```python
from build123d import *

# Parameters (mm, degrees)
SKETCH_1_R      = 2.125
SKETCH_1_R_2    = 8
EXTRUDE_1_DEPTH = 6


with BuildPart() as part:
    # 草图1 → 凸台-拉伸1 (new body)
    with BuildSketch(Plane.XY):
        with BuildLine():
            Line((-22.390026272, -12.434766873), (21.159720544, -12.434766873))
            ThreePointArc((21.159720544, -12.434766873), (27.298604017, -11.469317294), (32.844809242, -8.666177844))
            Line((32.844809242, -8.666177844), (77.295062426, 23.333822156))
            ThreePointArc((77.295062426, 23.333822156), (83.410279539, 30.44661958), (85.609973728, 39.565233127))
            Line((85.609973728, 39.565233127), (85.609973728, 149.565233127))
            Line((85.609973728, 149.565233127), (35.609973728, 149.565233127))
            Line((35.609973728, 149.565233127), (35.609973728, 39.565233127))
            Line((35.609973728, 39.565233127), (27.609973728, 39.565233127))
            Line((27.609973728, 39.565233127), (-22.390026272, 39.565233127))
            Line((-22.390026272, 39.565233127), (-22.390026272, -12.434766873))
        make_face()
        with Locations((-12.390026272, -2.434766873)):
            Circle(SKETCH_1_R, mode=Mode.SUBTRACT)
        with Locations((-4.390026272, -2.434766873)):
            Circle(SKETCH_1_R, mode=Mode.SUBTRACT)
        with Locations((19.609973728, -2.434766873)):
            Circle(SKETCH_1_R, mode=Mode.SUBTRACT)
        with Locations((-12.390026272, 29.565233127)):
            Circle(SKETCH_1_R, mode=Mode.SUBTRACT)
        with Locations((-4.390026272, 29.565233127)):
            Circle(SKETCH_1_R, mode=Mode.SUBTRACT)
        with Locations((19.609973728, 29.565233127)):
            Circle(SKETCH_1_R, mode=Mode.SUBTRACT)
        with Locations((3.609973728, 13.565233127)):
            Circle(SKETCH_1_R_2, mode=Mode.SUBTRACT)
        with BuildLine():
            Line((54.859973728, 92.565233127), (54.859973728, 62.565233127))
            ThreePointArc((54.859973728, 62.565233127), (50.609973728, 58.315233127), (46.359973728, 62.565233127))
            Line((46.359973728, 62.565233127), (46.359973728, 92.565233127))
            ThreePointArc((46.359973728, 92.565233127), (50.609973728, 96.815233127), (54.859973728, 92.565233127))
        make_face(mode=Mode.SUBTRACT)
        with BuildLine():
            Line((66.359973728, 109.565233127), (66.359973728, 139.565233127))
            ThreePointArc((66.359973728, 139.565233127), (70.609973728, 143.815233127), (74.859973728, 139.565233127))
            Line((74.859973728, 139.565233127), (74.859973728, 109.565233127))
            ThreePointArc((74.859973728, 109.565233127), (70.609973728, 105.315233127), (66.359973728, 109.565233127))
        make_face(mode=Mode.SUBTRACT)
    extrude(amount=EXTRUDE_1_DEPTH)


solid = part.part
```
Design review of the part built by this model. Coordinates are the model's own, in mm. A direction names the side the tool comes from. Round coordinates to 2 decimals unless told otherwise and drop trailing zeros. Order: outer loops, then holes, each group sorted by start corner. A loop starts at its lowest first (then second) coordinate and runs counter-clockwise, first axis right, second up. Notation, with made-up numbers: (-4, 31) - (52, 31) arc R25 ccw to (52, 45) - close; hole circle Ø5 at (-24.5, 70). An arc over 180 degrees is marked (long way). One line per question, with ' | ' between items.
Item 1: Wall thickness on line 1 (X direction, y = 68.5, z = 5.7); line 2 (Y direction, x = -5.5, z = 4.9); line 3 (Y direction, x = 3, z = 0.4): over which ranges is each line inside the solid? List them lowest first. Write a range as [from, to].
Checks:
line 1: [35.61, 46.36], [54.86, 85.61] | line 2: [-12.43, -4.25], [-0.62, 27.75], [31.38, 39.57] | line 3: [-12.43, 5.59], [21.54, 39.57]
Item 2: Machinability: for faces 4 (the face through (7, 39.565, 3)), 5 (the face through (46.36, 77, 3)), 6 (the face through (-1, -12.435, 3)), which of the approach directions +Z, -Z, +X, -X, +Y, -Y give a long, thin tool a straight path to every point of the face, cutting with its end or side? Answer none if there is none.
Checks:
face 4: +Z, -Z, -X, +Y | face 5: +Z, -Z | face 6: +Z, -Z, +X, -X, -Y
Item 3: Take a section at D-D, the plane y = 101.5. Write out the cut boundary in (x, z), then the cut area to 3 significant figures.
Checks:
outline: (35.61, 0) - (85.61, 0) - (85.61, 6) - (35.61, 6) - close | area: 300 mm²
Item 4: Draft analysis for pull direction X (two halves, no side actions). For faces 1 (the face through (20.59, 27.68, 2.96)), 2 (the face through (61, 149.565, 3)), 3 (the face through (54.76, 7.11, 2.96)), state which applies: +X half, -X half, draft (parallel to the pull), parting line (faces both ways), or undercut.
Checks:
face 1: undercut | face 2: draft | face 3: +X half
Item 5: Take a section at C-C, the plane z = 3.05. Give the number of separate pieces and of enclosed holes in the cut face, then the cut area to 3 significant figures.
Checks:
separate pieces: 1 | enclosed holes: 9 | area: 8,980 mm²
Item 6: Take a section at A-A, the plane y = 132. Write out the cut boundary in (x, z), then the cut area to 3 significant figures.
Checks:
outline: (35.61, 0) - (66.36, 0) - (66.36, 6) - (35.61, 6) - close; (74.86, 0) - (85.61, 0) - (85.61, 6) - (74.86, 6) - close | area: 249 mm²
Item 7: Take a section at B-B, the plane x = 3. Write out the cut boundary in (y, z).
Checks:
outline: (-12.43, 0) - (5.59, 0) - (5.59, 6) - (-12.43, 6) - close; (21.54, 0) - (39.57, 0) - (39.57, 6) - (21.54, 6) - close
Item 8: For P1, Ø4, axis at x = -4.39, y = -2.43, coming from the -Z side; P2, Ø5, axis at x = -12.39, y = -2.43, coming from the +Z side; P3, Ø1, axis at y = 37.5, z = 1.5, coming from the +X side; P4, Ø3, axis at y = 55.5, z = 1.5, coming from the -X side, all flat-tipped, find the tip position at first contact; note any pin that passes through.
Checks:
P1: through | P2: z = 6 | P3: x = 85.55 | P4: x = 35.61
